Read the model definition and answer for the solid it produces. Units are mm, in the model's axes. Face numbers are marked on the shaded views. Coordinates: 2 decimals unless noted, no trailing zeros. Order: outer loops, then holes, each group sorted by start corner. A loop starts at its lowest first (then second) coordinate and runs counter-clockwise, first axis right, second up. Notation, with made-up numbers: M -28.75,66.25 L -18.75,66.25 A25 cw -18.75,104.25 Z; hole C 52.5,-16 d4. An arc over 180 degrees is marked long. Use a Markdown table: item, result. Add a question column.
1) Find section A-A on x = 42. Write down the section's boundary in (y, z), plus the area to 3 significant figures.
2) Find the intervals of material crossed by probe 1 along Z at (x, y) = (-18, -1.1); probe 2 along Z at (x, y) = (-54, -0.6); probe 3 along Z at (x, y) = (16, -2.4), in increasing order. Write a range as [from, to].
3) The mould has two halves that part along Y. Classify the marked faces 1 and 2: released by +Y, released by -Y, zero draft, split by the parting line, or undercut.
4) Each of these flat-tipped pins is pushed along its axis until it touches: pin 1 Ø1.5 at (y, z) = (-1.5, 29) entering from +X; pin 2 Ø2.5 at (x, z) = (30, -2) entering from +Y; pin 3 Ø1.5 at (x, y) = (83, -2) entering from -Z; pin 4 Ø1.5 at (x, y) = (-41.5, -1) entering from +Z. Where does it stop, or does it pass through?
5) Find section B-B on y = -0.9. Count the separate pieces of the cut face and the enclosed holes in it, plus the area to 3 significant figures.
6) Find section C-C on z = -27. Write down the section's boundary in (x, y).
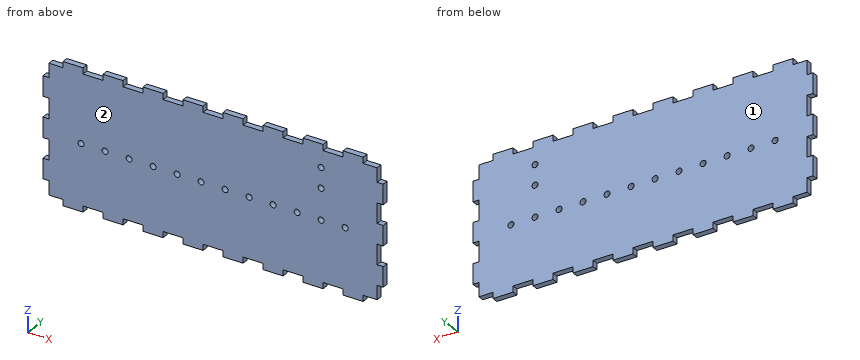
from build123d import *

# Parameters (mm, degrees)
F0_W     = 170
F0_H     = 70
F1_DEPTH = 3
F2_R     = 1.5
F3_DEPTH = 3.001
F4_R     = 1.5
F5_DEPTH = 3.001
F6_W     = 3
F6_H     = 3
F6_W_2   = 7
F6_W_3   = 10
F6_H_2   = 7
F7_DEPTH = 3.001


with BuildPart() as f1:
    # F0 (on Front) → F1 (new body)
    with BuildSketch(Plane.XZ):
        Rectangle(F0_W, F0_H)
    extrude(amount=F1_DEPTH)

    # F2 (on face) → F3 (cut, through all)
    with BuildSketch(Plane.XZ.offset(3)):
        with Locations((-66, -2)):
            Circle(F2_R)
        with Locations((-54, -2)):
            Circle(F2_R)
        with Locations((-42, -2)):
            Circle(F2_R)
        with Locations((-30, -2)):
            Circle(F2_R)
        with Locations((-18, -2)):
            Circle(F2_R)
        with Locations((-6, -2)):
            Circle(F2_R)
        with Locations((6, -2)):
            Circle(F2_R)
        with Locations((18, -2)):
            Circle(F2_R)
        with Locations((30, -2)):
            Circle(F2_R)
        with Locations((42, -2)):
            Circle(F2_R)
        with Locations((54, -2)):
            Circle(F2_R)
        with Locations((66, -2)):
            Circle(F2_R)
    extrude(amount=-F3_DEPTH, mode=Mode.SUBTRACT)

    # F4 (on face) → F5 (cut, through all)
    with BuildSketch(Plane.XZ.offset(3)):
        with Locations((54, 13.5)):
            Circle(F4_R)
        with Locations((54, 23.5)):
            Circle(F4_R)
    extrude(amount=-F5_DEPTH, mode=Mode.SUBTRACT)

    # F6 (on face) → F7 (cut, through all)
    with BuildSketch(Plane.XZ.offset(3)):
        with Locations((-83.5, -33.5)):
            Rectangle(F6_W, F6_H)
        with Locations((-78.5, -33.5)):
            Rectangle(F6_W_2, F6_H)
        Polygon((-85, -28), (-85, -32), (-82, -32), (-82, -25), (-85, -25), align=None)
        with Locations((-60, -33.5)):
            Rectangle(F6_W_3, F6_H)
        with Locations((-40, -33.5)):
            Rectangle(F6_W_3, F6_H)
        with Locations((-20, -33.5)):
            Rectangle(F6_W_3, F6_H)
        with Locations((0, -33.5)):
            Rectangle(F6_W_3, F6_H)
        with Locations((20, -33.5)):
            Rectangle(F6_W_3, F6_H)
        with Locations((40, -33.5)):
            Rectangle(F6_W_3, F6_H)
        with Locations((60, -33.5)):
            Rectangle(F6_W_3, F6_H)
        with Locations((83.5, -33.5)):
            Rectangle(F6_W, F6_H)
        Polygon((82, -32), (85, -32), (85, -28), (85, -25), (82, -25), align=None)
        with Locations((78.5, -33.5)):
            Rectangle(F6_W_2, F6_H)
        with Locations((-60, 33.5)):
            Rectangle(F6_W_3, F6_H)
        with Locations((-20, 33.5)):
            Rectangle(F6_W_3, F6_H)
        with Locations((-40, 33.5)):
            Rectangle(F6_W_3, F6_H)
        with Locations((0, 33.5)):
            Rectangle(F6_W_3, F6_H)
        with Locations((-83.5, 33.5)):
            Rectangle(F6_W, F6_H)
        with Locations((-83.5, 28.5)):
            Rectangle(F6_W, F6_H_2)
        with Locations((-78.5, 33.5)):
            Rectangle(F6_W_2, F6_H)
        with Locations((78.5, 33.5)):
            Rectangle(F6_W_2, F6_H)
        with Locations((83.5, 33.5)):
            Rectangle(F6_W, F6_H)
        with Locations((83.5, 28.5)):
            Rectangle(F6_W, F6_H_2)
        with Locations((20, 33.5)):
            Rectangle(F6_W_3, F6_H)
        with Locations((40, 33.5)):
            Rectangle(F6_W_3, F6_H)
        with Locations((60, 33.5)):
            Rectangle(F6_W_3, F6_H)
        Polygon((-82, 5), (-82, 15), (-85, 15), (-85, 12), (-85, 5), align=None)
        Polygon((-82, -15), (-82, -5), (-85, -5), (-85, -8), (-85, -15), align=None)
        Polygon((85, 12), (85, 15), (82, 15), (82, 5), (85, 5), align=None)
        Polygon((85, -8), (85, -5), (82, -5), (82, -15), (85, -15), align=None)
    extrude(amount=-F7_DEPTH, mode=Mode.SUBTRACT)


solid = f1.part
Check result:
| question | item | result |
|---|---|---|
| 1 | outline | M -3,-32 L 0,-32 L 0,-3.5 L -3,-3.5 Z; M -3,-0.5 L 0,-0.5 L 0,32 L -3,32 Z |
| 1 | area | 183 mm2 |
| 2 | probe 1 | z = [-32, -3.5], [-0.5, 32] |
| 2 | probe 2 | z = [-35, -3.5], [-0.5, 35] |
| 2 | probe 3 | z = [-32, 32] |
| 3 | face 1 | released by +Y |
| 3 | face 2 | released by -Y |
| 4 | pin 1 | stops at x = 82 |
| 4 | pin 2 | passes through |
| 4 | pin 3 | stops at z = -25 |
| 4 | pin 4 | stops at z = 32 |
| 5 | separate pieces | 1 |
| 5 | enclosed holes | 14 |
| 5 | area | 11,100 mm2 |
| 6 | outline | M -82,-3 L 82,-3 L 82,0 L -82,0 Z |
